```python
from build123d import *

# Parameters (mm, degrees)
SKETCH1_R           = 17.78
BOSS_EXTRUDE1_DEPTH = 11.049
SHELL1_T            = -1.27
SKETCH2_R           = 6.985
CUT_EXTRUDE1_DEPTH  = 27.97935583


with BuildPart() as part:
    # Sketch1 → Boss-Extrude1 (new body)
    with BuildSketch(Plane(origin=(0, 0, 0), x_dir=(1, 0, 0), z_dir=(0, 1, 0))):
        with Locations(Location((0, 0, 0), (0, 0, 270))):
            Circle(SKETCH1_R)
    extrude(amount=BOSS_EXTRUDE1_DEPTH)

    # Shell1
    shell1_openings = [part.faces().sort_by_distance(p)[0] for p in [
        (0, 11.049, 0),
    ]]
    offset(amount=SHELL1_T, openings=shell1_openings, kind=Kind.INTERSECTION)

    # Sketch2 → Cut-Extrude1 (cut, through all)
    with BuildSketch(Plane(origin=(0, 1.27, 0), x_dir=(1, 0, 0), z_dir=(0, 1, 0))):
        with Locations(Location((0, 0, 0), (0, 0, 270))):
            Circle(SKETCH2_R)
    extrude(amount=-CUT_EXTRUDE1_DEPTH, mode=Mode.SUBTRACT)


solid = part.part
```
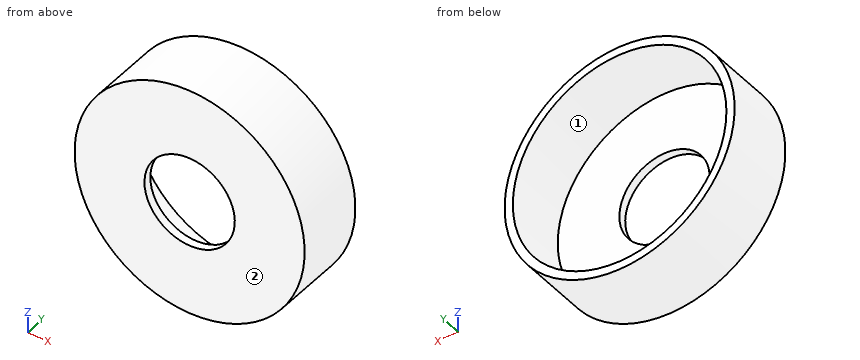
Verification items for the finished model (mm, model axes). Face numbers are marked on the shaded views. A direction names the side the tool comes from. Round coordinates to 2 decimals unless told otherwise and drop trailing zeros. Order: outer loops, then holes, each group sorted by start corner. A loop starts at its lowest first (then second) coordinate and runs counter-clockwise, first axis right, second up. Notation, with made-up numbers: (-35, -20.75) - (22, -20.75) arc R25 cw to (22, 3.25) - close; hole circle Ø2 at (25, -34.75). An arc over 180 degrees is marked (long way). Use CSV: the item, a comma, the result in double quotes. Start each with the question number.
1) Section check D-D, the plane y = 4. Record the cut outline in (x, z), plus the area to 3 significant figures.
2) Go/stop test with flat-tipped pins: P1, Ø4, axis at x = 8.5, y = 2.5, coming from the -Z side; P2, Ø5, axis at y = 10, z = 3, coming from the +X side; P3, Ø1, axis at y = 7.5, z = 5, coming from the +X side; P4, Ø8.5, axis at x = 0, z = 0, coming from the +Y side. Record where each tip stops, or that it passes through.
3) Thickness scan on L1, parallel to Z at x = -0.5, y = 5; L2, parallel to X at y = 8.25, z = 0; L3, parallel to X at y = 0.7, z = 0 (3 decimals). Record the ranges inside material, lowest first.
4) Section check B-B, the plane z = 0. Record the cut outline in (x, y) (3 decimals).
5) Section check C-C, the plane z = -10. Record the cut outline in (x, y), plus the area to 3 significant figures.
6) Access from +Z, -Z, +X, -X, +Y, -Y to the whole of each face (thin tool, end or side, straight path). Record for the marked faces 1 and 2.
7) Section check A-A, the plane x = 0. Record the cut outline in (y, z) (3 decimals).
Answers:
1,outline,"circle Ø35.56 at (0, 0); hole circle Ø33.02 at (0, 0)"
1,area,"137 mm²"
2,P1,"stops at z = -16.55"
2,P2,"stops at x = 17.77"
2,P3,"stops at x = 17.2"
2,P4,"passes through"
3,L1,"z = -17.77 to -16.5, 16.5 to 17.77"
3,L2,"x = -17.78 to -16.51, 16.51 to 17.78"
3,L3,"x = -17.78 to -6.985, 6.985 to 17.78"
4,outline,"(-17.78, 0) - (-6.985, 0) - (-6.985, 1.27) - (-16.51, 1.27) - (-16.51, 11.049) - (-17.78, 11.049) - close; (6.985, 0) - (17.78, 0) - (17.78, 11.049) - (16.51, 11.049) - (16.51, 1.27) - (6.985, 1.27) - close"
5,outline,"(-14.7, 0) - (14.7, 0) - (14.7, 11.05) - (13.14, 11.05) - (13.14, 1.27) - (-13.14, 1.27) - (-13.14, 11.05) - (-14.7, 11.05) - close"
5,area,"67.9 mm²"
6,face 1,"+Y"
6,face 2,"+Z, -Z, +X, -X, -Y"
7,outline,"(0, -17.78) - (11.049, -17.78) - (11.049, -16.51) - (1.27, -16.51) - (1.27, -6.985) - (0, -6.985) - close; (0, 6.985) - (1.27, 6.985) - (1.27, 16.51) - (11.049, 16.51) - (11.049, 17.78) - (0, 17.78) - close"
